```python
from build123d import *

# Parameters (mm, degrees)
F0_W           = 101.6
F0_H           = 101.6
F1_DEPTH       = 101.6
F2_W           = 86.36
F2_H           = 86.36
F3_DEPTH       = 46.99
F3_TAPER       = 40
F4_W           = 86.36
F4_H           = 86.36
F5_DEPTH       = 46.99
F5_TAPER       = 40
F6_W           = 86.36
F6_H           = 86.36
F7_DEPTH       = 46.99
F7_TAPER       = 40
F8_W           = 86.36
F8_H           = 86.36
F9_DEPTH       = 46.99
F9_TAPER       = 40
F10_W          = 86.36
F10_H          = 86.36
F11_DEPTH      = 46.99
F11_TAPER      = 40
F12_W          = 86.36
F12_H          = 86.36
F13_DEPTH      = 46.99
F13_TAPER      = 40
F14_W          = 12.581416662
F14_H          = 12.581416662
F15_DEPTH      = 2.54
F15_DEPTH_BACK = 10.16


with BuildPart() as f1:
    # F0 (on Top) → F1 (new body)
    with BuildSketch(Plane.XY):
        with Locations((-50.8, 50.8)):
            Rectangle(F0_W, F0_H)
    extrude(amount=F1_DEPTH)

    # F2 (on face) → F3 (cut)
    with BuildSketch(Plane.XZ):
        with Locations((-50.8, 50.8)):
            Rectangle(F2_W, F2_H)
    extrude(amount=-F3_DEPTH, taper=F3_TAPER, mode=Mode.SUBTRACT)

    # F4 (on face) → F5 (cut)
    with BuildSketch(Plane.YZ):
        with Locations((50.8, 50.8)):
            Rectangle(F4_W, F4_H)
    extrude(amount=-F5_DEPTH, taper=F5_TAPER, mode=Mode.SUBTRACT)

    # F6 (on face) → F7 (cut)
    with BuildSketch(Plane.XY.offset(101.6)):
        with Locations((-50.8, 50.8)):
            Rectangle(F6_W, F6_H)
    extrude(amount=-F7_DEPTH, taper=F7_TAPER, mode=Mode.SUBTRACT)

    # F8 (on face) → F9 (cut)
    with BuildSketch(Plane(origin=(-101.6, 0, 0), x_dir=(0, -1, 0), z_dir=(-1, 0, 0))):
        with Locations((-50.8, 50.8)):
            Rectangle(F8_W, F8_H)
    extrude(amount=-F9_DEPTH, taper=F9_TAPER, mode=Mode.SUBTRACT)

    # F10 (on face) → F11 (cut)
    with BuildSketch(Plane(origin=(0, 101.6, 0), x_dir=(-1, 0, 0), z_dir=(0, 1, 0))):
        with Locations((50.8, 50.8)):
            Rectangle(F10_W, F10_H)
    extrude(amount=-F11_DEPTH, taper=F11_TAPER, mode=Mode.SUBTRACT)

    # F12 (on face) → F13 (cut)
    with BuildSketch(Plane(origin=(0, 0, 0), x_dir=(1, 0, 0), z_dir=(0, 0, -1))):
        with Locations((-50.8, -50.8)):
            Rectangle(F12_W, F12_H)
    extrude(amount=-F13_DEPTH, taper=F13_TAPER, mode=Mode.SUBTRACT)

    # F14 (on face) → F15 (join, two sides)
    with BuildSketch(Plane.XZ.offset(-46.99)) as f15_sk:
        with Locations((-50.8, 50.8)):
            Rectangle(F14_W, F14_H)
    extrude(amount=F15_DEPTH)
    extrude(f15_sk.sketch, amount=-F15_DEPTH_BACK)


solid = f1.part
```
Geometry check sheet. Reference: the model listing, model coordinates, mm. A direction names the side the tool comes from. Coordinates: 2 decimals unless noted, no trailing zeros. One line per question, with ' | ' between items. Start each with the question number.
Item 1: Material ranges on L1, parallel to X at y = 23, z = 66; L2, parallel to Z at x = -51, y = 9; L3, parallel to X at y = 79.5, z = 10.5, recorded low to high. Write a range as [from, to].
Item 2: Gauge pin test, flat ends, axial feed: pin 1 (1.5 mm diameter, centred on y = 40, z = 81, fed in from -X); pin 2 (3 mm diameter, centred on y = 48.5, z = 42.5, fed in from +X); pin 3 (9.5 mm diameter, centred on x = -48, y = 49, fed in from -Z). Record the tip position at first contact, or that the pin passes through.
Item 3: Set-up check for faces 1 (the flat face through (-57.091, 51, 51)), 2 (the flat face through (-51, 51, 44.509)), 3 (the flat face through (-51, 51, 57.091)), 4 (the flat face through (-6, 52, 101.6)), 5 (the flat face through (-51, 44.45, 51)): record each of +Z, -Z, +X, -X, +Y, -Y from which the full face is reachable in a straight line by a thin tool's end or side.
Item 4: Draft check along Z on faces 6 (the flat face through (-51, 57.15, 51)), 7 (the flat face through (-6, 52, 0)), 8 (the flat face through (-44.509, 51, 51)), 9 (the flat face through (0, 95, 50)). Enter one of: pulls with the +Z half, pulls with the -Z half, needs draft (parallel to the pull), parting line crosses it, or undercut.
Findings:
1) L1: x = [-83.27, -74.68], [-26.92, -18.33] | L2: z = [1.64, 15.17], [86.43, 99.96] | L3: x = [-98.17, -85.17], [-16.43, -3.43]
2) pin 1: stops at x = -87.02 | pin 2: stops at x = -39.78 | pin 3: stops at z = 42.46
3) face 1: -X | face 2: -Z | face 3: +Z | face 4: +Z, +X, -X, +Y, -Y | face 5: -Y
4) face 6: undercut | face 7: pulls with the -Z half | face 8: undercut | face 9: needs draft
